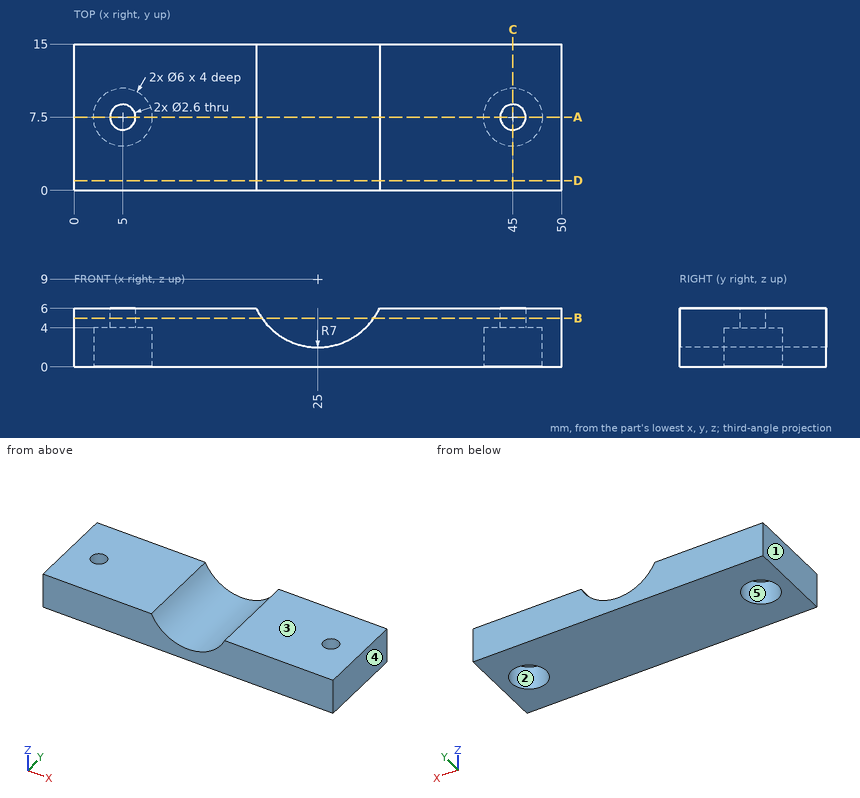
The drawing under review shows one solid part. Ordinate dimensions are in mm from its lowest x, y, z. A direction names the side the tool comes from. Give positions to 0.01 mm unless a question says otherwise; leave off trailing zeros. Order: outer loops, then holes, each group sorted by start corner. A loop starts at its lowest first (then second) coordinate and runs counter-clockwise, first axis right, second up. Notation, with made-up numbers: (32, 47.5) -> (62, 47.5) arc R13 ccw to (62, 51.5) -> close; hole circle Ø2 at (13, 8.25). An arc over 180 degrees is marked (long way). Write item = value, one per line. Start each with the question number.
(1) To check wall thickness, follow line 1 along X through (y, z) = (7.5, 0.95); line 2 along Y through (x, z) = (5, 1.4); line 3 along Y through (x, z) = (5, 5.1). State the ranges of each line that lie inside material, in increasing order.
(2) For the marked faces 4 and 5, list the 3-axis set-ups (+Z, -Z, +X, -X, +Y, -Y) from which the entire face can be reached by the end or side of a thin tool; tool diameter is ignored.
(3) Mouldability with a two-part tool opening along X and no side actions: class the marked faces 1, 2 and 3 as +X half, -X half, draft (parallel to the pull), parting line (faces both ways), or undercut.
(4) We need section B-B on z = 5. Write out the cut boundary in (x, y), plus the area to 3 significant figures.
(5) We need section D-D on y = 1. Write out the cut boundary in (x, z).
(6) We need section A-A on y = 7.5. Write out the cut boundary in (x, z), plus the area to 3 significant figures.
(7) We need section C-C on x = 45. Write out the cut boundary in (y, z).
(8) For pin 1 (2.5 mm diameter, centred on x = 5, y = 7.5, fed in from -Z); pin 2 (1 mm diameter, centred on x = 22, y = 3, fed in from +Z); pin 3 (1.8 mm diameter, centred on x = 4.5, y = 7.5, fed in from -Z), all flat-tipped, find the tip position at first contact; note any pin that passes through.
Numbers:
q1.line_1 = 0 to 2, 8 to 42, 48 to 50
q1.line_2 = 0 to 4.5, 10.5 to 15
q1.line_3 = 0 to 6.2, 8.8 to 15
q2.face_4 = +Z, -Z, +X, +Y, -Y
q2.face_5 = -Z
q3.face_1 = -X half
q3.face_2 = undercut
q3.face_3 = draft
q4.outline = (0, 0) -> (19.26, 0) -> (19.26, 15) -> (0, 15) -> close; (30.74, 0) -> (50, 0) -> (50, 15) -> (30.74, 15) -> close; hole circle Ø2.6 at (5, 7.5); hole circle Ø2.6 at (45, 7.5)
q4.area = 567 mm^2
q5.outline = (0, 0) -> (50, 0) -> (50, 6) -> (31.32, 6) arc R7 cw to (18.68, 6) -> (0, 6) -> close
q6.outline = (0, 0) -> (2, 0) -> (2, 4) -> (3.7, 4) -> (3.7, 6) -> (0, 6) -> close; (6.3, 4) -> (8, 4) -> (8, 0) -> (42, 0) -> (42, 4) -> (43.7, 4) -> (43.7, 6) -> (31.32, 6) arc R7 cw to (18.68, 6) -> (6.3, 6) -> close; (46.3, 4) -> (48, 4) -> (48, 0) -> (50, 0) -> (50, 6) -> (46.3, 6) -> close
q6.area = 205 mm^2
q7.outline = (0, 0) -> (4.5, 0) -> (4.5, 4) -> (6.2, 4) -> (6.2, 6) -> (0, 6) -> close; (8.8, 4) -> (10.5, 4) -> (10.5, 0) -> (15, 0) -> (15, 6) -> (8.8, 6) -> close
q8.pin_1 = through
q8.pin_2 = 2.94
q8.pin_3 = 4
